Autodesk Inventor part; units mm, degrees
ref_plane "YZ Plane" through (0, 0, 0) normal (1, 0, 0) x (0, 1, 0)
ref_plane "XZ Plane" through (0, 0, 0) normal (0, 1, 0) x (-1, 0, 0)
ref_plane "XY Plane" through (0, 0, 0) normal (0, 0, 1) x (1, 0, 0)
sketch "Sketch1" plane through (0, 0, 0) normal (0, 0, 1) x (1, 0, 0)
  line L0 (0, -17.78) -> (0, 106.68)
  line L1 (66.675, 88.9) -> (66.675, 0)
  line L2 (66.675, 0) -> (-66.675, 0)
  line L3 (-66.675, 0) -> (-66.675, 88.9)
  line L4 (-93.345, 0) -> (93.345, 0)
  line L5 (-12.7, 88.9) -> (-12.7, 63.5)
  line L6 (-12.7, 63.5) -> (12.7, 63.5)
  line L7 (12.7, 63.5) -> (12.7, 88.9)
  line L8 (-66.675, 88.9) -> (-12.7, 88.9)
  line L9 (12.7, 88.9) -> (66.675, 88.9)
  line L10 (0, 0) -> (0, 26.797)
  circle A0 centre (0, 26.797) radius 14.2875
  dimension "d0" = 133.35
  dimension "d1" = 88.9
  dimension "d2" = 25.4
  dimension "d3" = 25.4
  dimension "d5" = 28.575
  dimension "d19" = 62.103
extrude "Extrusion1" add sketch "Sketch1" along normal blind 3.175 contours L2 L3 L8 L5 L6 L0 A0 | L0 A0 L6 L7 L9 L1 L2
sketch "Sketch2" plane through (0, 0, 3.175) normal (0, 0, 1) x (1, 0, 0)
  line L0 (66.675, 0) -> (66.675, 88.9)
  line L1 (-66.675, 0) -> (66.675, 0)
  line L2 (66.675, 88.9) -> (12.7, 88.9)
  point P0 (0, 0)
  point P1 (53.975, 69.85)
  point P2 (53.975, 19.05)
  dimension "d16" = 12.7
  dimension "d18" = 19.05
  dimension "d20" = 19.05
hole "Hole1" at (53.975, 69.85, 3.175) at (53.975, 19.05, 3.175) direction (0, 0, -1) diameter 5.5118 end through all
mirror "Mirror1" about plane through (0, 0, 0) normal (1, 0, 0) of "Hole1"
properties part number "DIFF_PLATE_ROD_SHORT"
The listing builds one solid part. Answer for the finished solid, in the listing's coordinates (mm). A direction names the side the tool comes from. Give positions to 0.01 mm unless a question says otherwise; leave off trailing zeros. Write each loop counter-clockwise with the first axis right and the second up, starting at its lowest first coordinate (ties: lowest second). Pieces come first, ordered by that corner, then holes.
1) Given P1, Ø1.6, axis at x = 4.5, z = 2, coming from the +Y side, flat-ended and moving along its own axis, determine where the tip first touches the part or whether it passes through.
2) Section B-B (y = 69.85) is taken. Write down the section's boundary in (x, z) (3 decimals).
3) Section A-A (y = 83.5) is taken. Write down the section's boundary in (x, z) (3 decimals), and give its area (3 significant figures).
4) Section C-C (x = 9.5) is taken. Write down the section's boundary in (y, z) (3 decimals).
5) A tool of negligible diameter and unlimited length cuts with its end or side. For faces 1 (the face through (51.243, 70.209, 1.565)), 2 (the face through (12.7, 76, 2)), from which of +Z, -Z, +X, -X, +Y, -Y can it reach the whole face along a straight path? Write none if from no direction.
6) Section D-D (z = 0.95) is taken. Count the separate pieces of the cut face and the enclosed holes in it, and give its area (3 significant figures).
7) For a pull along X with two mould halves and no side action, classify faces 3 (the face through (-3.097, 40.745, 1.565)), 4 (the face through (-1, 45, 3.175)), 5 (the face through (-66.675, 44, 2)), 6 (the face through (-51.285, 70.447, 1.565)) as pulls with the +X half, pulls with the -X half, needs draft (parallel to the pull), parting line crosses it, or undercut.
8) Find the intervals of material crossed by L1, parallel to X at y = 69.85, z = 1.7 (3 decimals); L2, parallel to X at y = 19.05, z = 2.25 (3 decimals); L3, parallel to X at y = 64, z = 2 (3 decimals), in increasing order.
Response:
1. P1: stops at y = 63.5
2. outline: (-66.675, 0) - (-56.731, 0) - (-56.731, 3.175) - (-66.675, 3.175) - close; (-51.219, 0) - (-12.7, 0) - (-12.7, 3.175) - (-51.219, 3.175) - close; (12.7, 0) - (51.219, 0) - (51.219, 3.175) - (12.7, 3.175) - close; (56.731, 0) - (66.675, 0) - (66.675, 3.175) - (56.731, 3.175) - close
3. outline: (-66.675, 0) - (-12.7, 0) - (-12.7, 3.175) - (-66.675, 3.175) - close; (12.7, 0) - (66.675, 0) - (66.675, 3.175) - (12.7, 3.175) - close
3. area: 343 mm2
4. outline: (0, 0) - (16.125, 0) - (16.125, 3.175) - (0, 3.175) - close; (37.469, 0) - (63.5, 0) - (63.5, 3.175) - (37.469, 3.175) - close
5. face 1: +Z, -Z
5. face 2: +Z, -Z, +Y
6. separate pieces: 1
6. enclosed holes: 5
6. area: 10,500 mm2
7. face 3: undercut
7. face 4: needs draft
7. face 5: pulls with the -X half
7. face 6: undercut
8. L1: x = -66.675 to -56.731, -51.219 to -12.7, 12.7 to 51.219, 56.731 to 66.675
8. L2: x = -66.675 to -56.731, -51.219 to -12.005, 12.005 to 51.219, 56.731 to 66.675
8. L3: x = -66.675 to -12.7, 12.7 to 66.675
